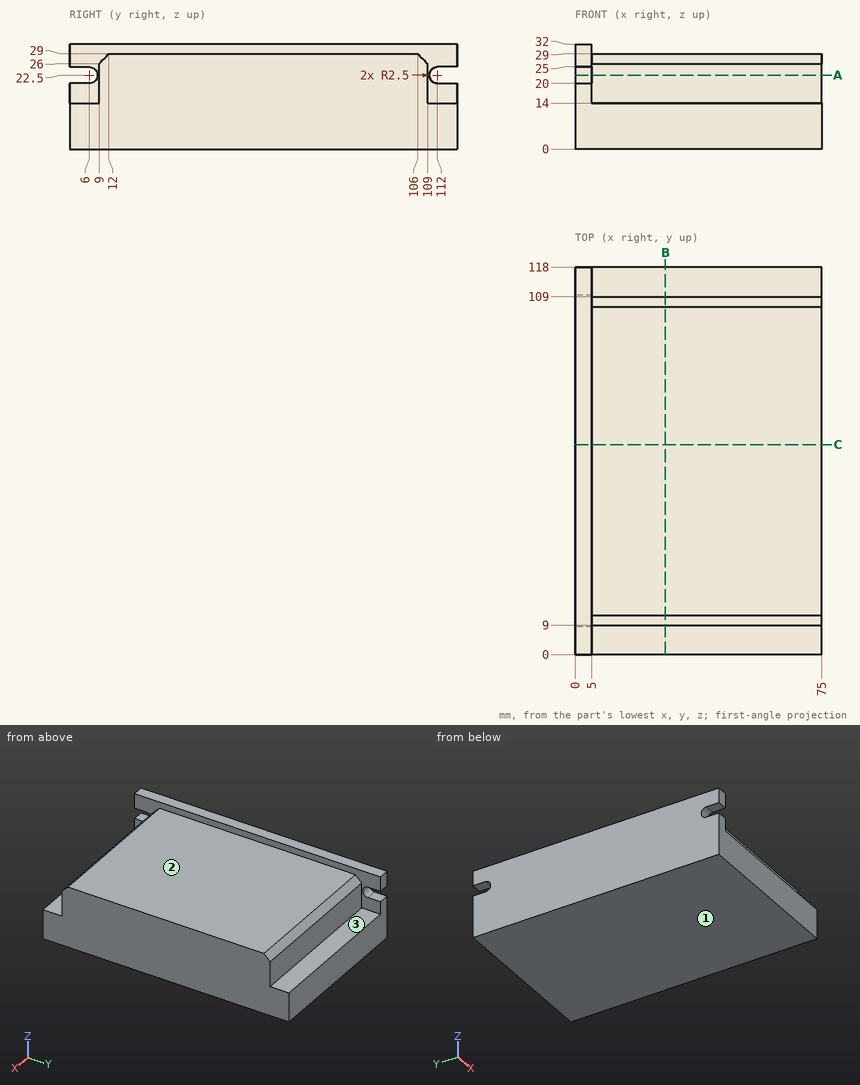
Geometry check sheet. Reference: drawing and pictorial views, mm from the part's lowest x, y, z. A direction names the side the tool comes from. Give positions to 0.01 mm unless a question says otherwise; leave off trailing zeros. Order: outer loops, then holes, each group sorted by start corner. A loop starts at its lowest first (then second) coordinate and runs counter-clockwise, first axis right, second up. Notation, with made-up numbers: M 31,3 L 70,3 A13 ccw 70,23 Z; hole C 7.5,-39.5 d7. An arc over 180 degrees is marked long. Answer in a Markdown table with one row per item.
1) Cross-section at C-C, the plane y = 64. Enter the section's corners in (x, z).
Filled sheet:
| item | result |
|---|---|
| outline | M 0,0 L 75,0 L 75,29 L 5,29 L 5,32 L 0,32 Z |
2) Access from +Z, -Z, +X, -X, +Y, -Y to the whole of each face (thin tool, end or side, straight path). Record for the marked faces 1, 2 and 3.
Filled sheet:
| item | result |
|---|---|
| face 1 | -Z, +X, -X, +Y, -Y |
| face 2 | +Z, +X, +Y, -Y |
| face 3 | +Z, +X, +Y |
3) Cross-section at A-A, the plane z = 22.5. Enter the section's corners in (x, y), plus the area to 4 significant figures.
Filled sheet:
| item | result |
|---|---|
| outline | M 0,8.5 L 5,8.5 L 5,9 L 75,9 L 75,109 L 5,109 L 5,109.5 L 0,109.5 Z |
| area | 7,505 mm2 |
4) Gauge pin test, flat ends, axial feed: P1, Ø1, axis at x = 24.5, y = 56, coming from the +Z side; P2, Ø4.5, axis at x = 52.5, y = 3, coming from the +Z side; P3, Ø7, axis at x = 25.5, y = 112, coming from the +Z side. Record the tip position at first contact, or that the pin passes through.
Filled sheet:
| item | result |
|---|---|
| P1 | stops at z = 29 |
| P2 | stops at z = 14 |
| P3 | stops at z = 26.5 |
5) Thickness scan on L1, parallel to Z at x = 64.5, y = 97; L2, parallel to Y at x = 28, z = 16.5; L3, parallel to Z at x = 70.5, y = 109.5. Record the ranges inside material, lowest first. Write a range as [from, to].
Filled sheet:
| item | result |
|---|---|
| L1 | z = [0, 29] |
| L2 | y = [9, 109] |
| L3 | z = [0, 14] |
6) Cross-section at B-B, the plane x = 27.5. Enter the section's corners in (y, z).
Filled sheet:
| item | result |
|---|---|
| outline | M 0,0 L 118,0 L 118,14 L 109,14 L 109,26 L 106,29 L 12,29 L 9,26 L 9,14 L 0,14 Z |
